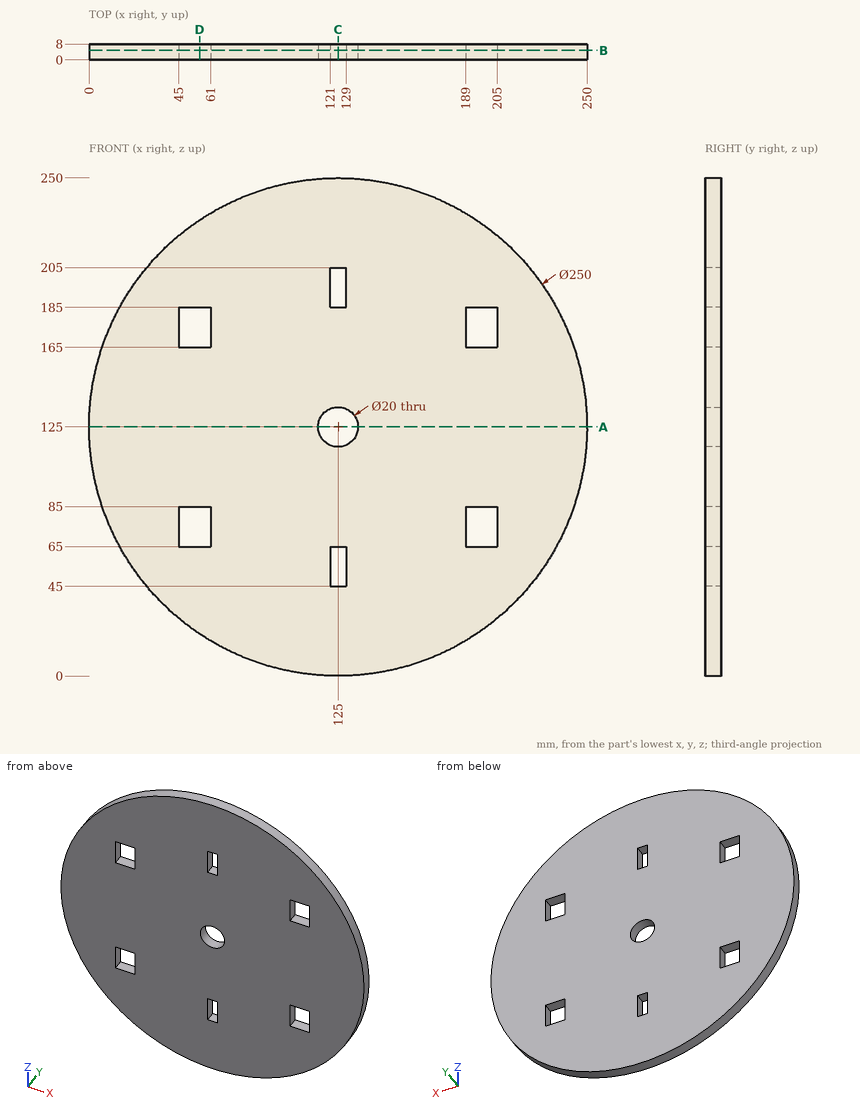
Drawing for the job (mm, zero at the part's lowest x, y, z). Give positions to 0.01 mm unless a question says otherwise; leave off trailing zeros. Order: outer loops, then holes, each group sorted by start corner. A loop starts at its lowest first (then second) coordinate and runs counter-clockwise, first axis right, second up. Notation, with made-up numbers: (-7.5, 34.5) -> (-3.5, 34.5) arc R22 cw to (-3.5, 46.5) -> close; hole circle Ø11 at (39.25, 2). An arc over 180 degrees is marked (long way). Use one line per item in the form item = value.
(1) Saw through at D-D (x = 55.5). Write the cut outline in (y, z).
Solution:
outline = (0, 21.1) -> (8, 21.1) -> (8, 65) -> (0, 65) -> close; (0, 85) -> (8, 85) -> (8, 165) -> (0, 165) -> close; (0, 185) -> (8, 185) -> (8, 228.9) -> (0, 228.9) -> close
(2) Saw through at A-A (z = 125). Write the cut outline in (x, y).
Solution:
outline = (0, 0) -> (115, 0) -> (115, 8) -> (0, 8) -> close; (135, 0) -> (250, 0) -> (250, 8) -> (135, 8) -> close
(3) Drill centre lines: line 1 (X direction, y = 6.25, z = 125); line 2 (X direction, y = 7.5, z = 68.5); line 3 (X direction, y = 7, z = 79.5). Where is each one in solid material? Low to high. Write a range as from..to.
Solution:
line_1 = 0..115, 135..250
line_2 = 13.5..45, 61..189, 205..236.5
line_3 = 8.58..45, 61..189, 205..241.42
(4) Saw through at B-B (y = 4.75). Write the cut outline in (x, z).
Solution:
outline = circle Ø250 at (125, 125); hole (45, 65) -> (61, 65) -> (61, 85) -> (45, 85) -> close; hole (45, 165) -> (61, 165) -> (61, 185) -> (45, 185) -> close; hole circle Ø20 at (125, 125); hole (121, 45) -> (129, 45) -> (129, 65) -> (121, 65) -> close; hole (121, 185) -> (129, 185) -> (129, 205) -> (121, 205) -> close; hole (189, 65) -> (205, 65) -> (205, 85) -> (189, 85) -> close; hole (189, 165) -> (205, 165) -> (205, 185) -> (189, 185) -> close
(5) Flat gauge pins, fed straight in: P1, Ø4, axis at x = 193.5, y = 2, coming from the -Z side; P2, Ø2.5, axis at x = 194, y = 4, coming from the +Z side; P3, Ø4, axis at y = 5.5, z = 77.5, coming from the +X side; P4, Ø4, axis at x = 124.5, y = 3.5, coming from the +Z side. Where does each tip first touch, or does it go through?
Solution:
P1 = 19.16
P2 = 230.05
P3 = 241.42
P4 = 250
(6) Saw through at C-C (x = 125). Write the cut outline in (y, z), then the cut area to 3 significant figures.
Solution:
outline = (0, 0) -> (8, 0) -> (8, 45) -> (0, 45) -> close; (0, 65) -> (8, 65) -> (8, 115) -> (0, 115) -> close; (0, 135) -> (8, 135) -> (8, 185) -> (0, 185) -> close; (0, 205) -> (8, 205) -> (8, 250) -> (0, 250) -> close
area = 1,520 mm²
